from build123d import *

# Parameters (mm, degrees)
F1_DEPTH    = 5
F2_R        = 1.1043953889
F3_DEPTH    = 5
F4_R        = 2.5
F5_T1_DEPTH = 20
F6_F1_R     = 1
F6_F2_R     = 1
F6_F3_R     = 0.9999
F6_F4_R     = 0.9996
F7_R        = 2.49999


# Not quite as in the source:
# - a fillet or chamfer that OpenCascade refuses, or shapes differently, is made with other operations: its cross-section is extruded or revolved along the edge and cut away or added
# - a fillet or chamfer is up to 0.001 mm smaller than in the source, because OpenCascade refuses the exact size


with BuildPart() as f1:
    # F0 (on Top) → F1 (new body)
    with BuildSketch(Plane.XY):
        with BuildLine():
            ThreePointArc((4.2426406871, 4.2426406871), (0, -6), (-4.2426406871, 4.2426406871))
            Line((-4.2426406871, 4.2426406871), (-6.0104076401, 6.0104076401))
            ThreePointArc((-6.0104076401, 6.0104076401), (-8.1830596791, -2.2994639132), (-2, -8.2613558209))
            Line((-2, -8.2613558209), (-2, -12.2613558209))
            Line((-2, -12.2613558209), (-1, -12.2613558209))
            Line((-1, -12.2613558209), (-1, -20.2613558209))
            Line((-1, -20.2613558209), (0, -20.2613558209))
            Line((0, -20.2613558209), (1, -20.2613558209))
            Line((1, -20.2613558209), (1, -12.2613558209))
            Line((1, -12.2613558209), (2, -12.2613558209))
            Line((2, -12.2613558209), (2, -8.2613558209))
            ThreePointArc((2, -8.2613558209), (8.1830596791, -2.2994639132), (6.0104076401, 6.0104076401))
            Line((6.0104076401, 6.0104076401), (4.2426406871, 4.2426406871))
        make_face()
    extrude(amount=F1_DEPTH)

    # F2 (on face) → F3 (cut)
    with BuildSketch(Plane(origin=(-1, 0, 0), x_dir=(0, -1, 0), z_dir=(-1, 0, 0))):
        with Locations((17.756960432, 2.4956046111)):
            Circle(F2_R)
    extrude(amount=-F3_DEPTH, mode=Mode.SUBTRACT)

    # F4
    f4_edges = [f1.edges().sort_by_distance(p)[0] for p in [
        (4.242641, 4.242641, 2.5),
        (-4.242641, 4.242641, 2.5),
    ]]
    fillet(f4_edges, radius=F4_R)

    # F5: fillet of radius 5 on 2 edges, made by hand

    # F5_s2 → F5_t1 (cut)
    with BuildSketch(Plane.XY.offset(-7.5)):
        with BuildLine():
            ThreePointArc((2, -9.2613558209), (1.7434164903, -10.842494651), (1, -12.2613558209))
            Line((1, -12.2613558209), (2, -12.2613558209))
            Line((2, -12.2613558209), (2, -9.2613558209))
        make_face()
        with BuildLine():
            ThreePointArc((-2, -9.2613558209), (-1.7434164903, -10.842494651), (-1, -12.2613558209))
            Line((-1, -12.2613558209), (-2, -12.2613558209))
            Line((-2, -12.2613558209), (-2, -9.2613558209))
        make_face()
    extrude(amount=F5_T1_DEPTH, mode=Mode.SUBTRACT)

    # F6: fillet of radius 1 on 6 edges, made by hand

    # F6_f1
    f6_f1_edges = [f1.edges().sort_by_distance(p)[0] for p in [
        (-2, -8.2613558209, 2.5),
    ]]
    fillet(f6_f1_edges, radius=F6_F1_R)

    # F6_f2
    f6_f2_edges = [f1.edges().sort_by_distance(p)[0] for p in [
        (2, -8.2613558209, 2.5),
    ]]
    fillet(f6_f2_edges, radius=F6_F2_R)

    # F6_f3 (radius 1 in the source; OpenCascade refuses exactly that, so slightly less here)
    f6_f3_edges = [f1.edges().sort_by_distance(p)[0] for p in [
        (2, -9.1376170048, 5),
        (1.7434164903, -10.842494651, 5),
    ]]
    fillet(f6_f3_edges, radius=F6_F3_R)

    # F6_f4 (radius 1 in the source; OpenCascade refuses exactly that, so slightly less here)
    f6_f4_edges = [f1.edges().sort_by_distance(p)[0] for p in [
        (-1.7434164903, -10.842494651, 5),
        (-2, -9.1376170048, 5),
    ]]
    fillet(f6_f4_edges, radius=F6_F4_R)

    # F7 (radius 2.5 in the source; OpenCascade refuses exactly that, so slightly less here)
    f7_edges = [f1.edges().sort_by_distance(p)[0] for p in [
        (0, -20.261356, 5),
        (0, -20.261356, 0),
    ]]
    fillet(f7_edges, radius=F7_R)


solid = f1.part
Design review of the part built by this model. Coordinates are the model's own, in mm. A direction names the side the tool comes from. Round coordinates to 2 decimals unless told otherwise and drop trailing zeros. Write each loop counter-clockwise with the first axis right and the second up, starting at its lowest first coordinate (ties: lowest second). Pieces come first, ordered by that corner, then holes. Notation, with made-up numbers: (-24, 28.25) - (-5, 28.25) arc R24 cw to (-5, 64.25) - close; hole circle Ø6 at (27.25, 73). An arc over 180 degrees is marked (long way). Use a Markdown table: item, result. Add a question column.
1. We need section C-C (z = 0.7). State the section outline as (x, y) points, then the cut area to 3 significant figures.
2. Wall thickness on probe 1 along X at (y, z) = (0, 3.5); probe 2 along X at (y, z) = (4, 3.5); probe 3 along Y at (x, z) = (0.5, 1.9): over which ranges is each line inside the solid? List them lowest first.
3. We need section A-A (z = 3.1). State the section outline as (x, y) points, then the cut area to 3 significant figures.
4. For faces 4 (the face through (5.037, 4.327, 2.535)), 5 (the face through (-1.75, -10.82, 1.97)), list the 3-axis set-ups (+Z, -Z, +X, -X, +Y, -Y) from which the entire face can be reached by the end or side of a thin tool; tool diameter is ignored.
5. Mouldability with a two-part tool opening along X and no side actions: class faces 1 (the face through (0, -6, 2)), 2 (the face through (0.014, -19.51, 0.713)), 3 (the face through (-8.3, -1.84, 1.97)) as +X half, -X half, draft (parallel to the pull), parting line (faces both ways), or undercut.
6. Clearance check with flat-ended pins moving along their axes: pin 1 (1 mm diameter, centred on y = 3.5, z = 0.5, fed in from -X); pin 2 (1.5 mm diameter, centred on y = -17, z = 4.5, fed in from +X); pin 3 (3 mm diameter, centred on y = 3, z = 2, fed in from +X). State where each tip first meets the part, or that it passes through.
7. We need section D-D (y = -16). State the section outline as (x, z) points, then the cut area to 3 significant figures.
Output:
| question | item | result |
|---|---|---|
| 1 | outline | (-6.01, 6.01) arc R8.5 ccw to (-2.68, -8.07) arc R1 cw to (-2, -9.01) - (-2, -9.26) arc R5 ccw to (-1, -12.26) - (-1, -19.5) - (1, -19.5) - (1, -12.26) arc R5 ccw to (2, -9.26) - (2, -9.01) arc R1 cw to (2.68, -8.07) arc R8.5 ccw to (6.01, 6.01) - (5.74, 5.74) arc R2.5 ccw to (5.3, 2.81) arc R6 cw (long way) to (-5.3, 2.81) arc R2.5 ccw to (-5.74, 5.74) - close |
| 1 | area | 112 mm2 |
| 2 | probe 1 | x = -8.5 to -6, 6 to 8.5 |
| 2 | probe 2 | x = -7.5 to -5.01, 5.01 to 7.5 |
| 2 | probe 3 | y = -20.19 to -18.69, -16.83 to -5.98 |
| 3 | outline | (-6.01, 6.01) arc R8.5 ccw to (-2.68, -8.07) arc R1 cw to (-2, -9.01) - (-2, -9.26) arc R5 ccw to (-1, -12.26) - (-1, -16.83) - (1, -16.83) - (1, -12.26) arc R5 ccw to (2, -9.26) - (2, -9.01) arc R1 cw to (2.68, -8.07) arc R8.5 ccw to (6.01, 6.01) - (5.74, 5.74) arc R2.5 ccw to (5.3, 2.81) arc R6 cw (long way) to (-5.3, 2.81) arc R2.5 ccw to (-5.74, 5.74) - close; (-1, -20.19) - (1, -20.19) - (1, -18.68) - (-1, -18.68) - close |
| 3 | area | 110 mm2 |
| 4 | face 4 | +Z, -Z |
| 4 | face 5 | +Z, -Z, -X, -Y |
| 5 | face 1 | undercut |
| 5 | face 2 | draft |
| 5 | face 3 | -X half |
| 6 | pin 1 | stops at x = -7.95 |
| 6 | pin 2 | stops at x = 1 |
| 6 | pin 3 | stops at x = 8.37 |
| 7 | outline | (-1, 0) - (1, 0) - (1, 5) - (-1, 5) - close |
| 7 | area | 10.0 mm2 |
